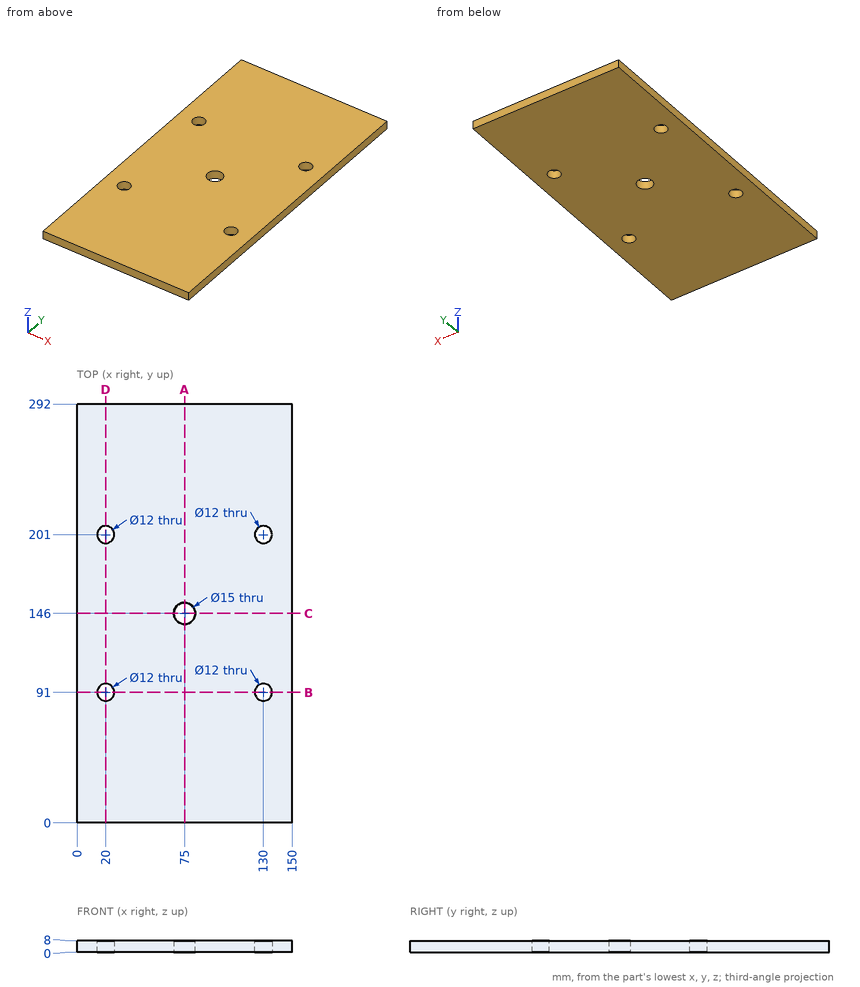
Input: dimensioned drawing with shaded views. Units: mm. Origin: part minimum x, y, z. Coordinates: 2 decimals unless noted, no trailing zeros. Loops run counter-clockwise (first coordinate to the right, second up) from the corner with the lowest first, then second, coordinate; pieces in that order, holes last. Notation, with made-up numbers: (76, -11) -> (106, -11) arc R16 cw to (106, 4) -> close; hole circle Ø10 at (31.25, -12). An arc over 180 degrees is marked (long way). Use a Markdown table: item, result. Add a question column.
(1) Section query B-B, the plane y = 91. Return loops of the section in (x, z), plus the area to 3 significant figures.
(2) Line query: line 1 along Y through (x, z) = (20, 4.5); line 2 along Y through (x, z) = (72, 1). Output: solid intervals per line, ascending.
(3) Section query D-D, the plane x = 20. Return loops of the section in (y, z), plus the area to 3 significant figures.
(4) Section query A-A, the plane x = 75. Return loops of the section in (y, z), plus the area to 3 significant figures.
(5) Section query C-C, the plane y = 146. Return loops of the section in (x, z).
(6) Pin query (flat end, axial travel): pin 1 Ø11 at (x, y) = (130, 91) entering from +Z. Return the tip coordinate at first contact, or that it passes through.
Answer:
| question | item | result |
|---|---|---|
| 1 | outline | (0, 0) -> (14, 0) -> (14, 8) -> (0, 8) -> close; (26, 0) -> (124, 0) -> (124, 8) -> (26, 8) -> close; (136, 0) -> (150, 0) -> (150, 8) -> (136, 8) -> close |
| 1 | area | 1,010 mm^2 |
| 2 | line 1 | y = 0 to 85, 97 to 195, 207 to 292 |
| 2 | line 2 | y = 0 to 139.13, 152.87 to 292 |
| 3 | outline | (0, 0) -> (85, 0) -> (85, 8) -> (0, 8) -> close; (97, 0) -> (195, 0) -> (195, 8) -> (97, 8) -> close; (207, 0) -> (292, 0) -> (292, 8) -> (207, 8) -> close |
| 3 | area | 2,140 mm^2 |
| 4 | outline | (0, 0) -> (138.5, 0) -> (138.5, 8) -> (0, 8) -> close; (153.5, 0) -> (292, 0) -> (292, 8) -> (153.5, 8) -> close |
| 4 | area | 2,220 mm^2 |
| 5 | outline | (0, 0) -> (67.5, 0) -> (67.5, 8) -> (0, 8) -> close; (82.5, 0) -> (150, 0) -> (150, 8) -> (82.5, 8) -> close |
| 6 | pin 1 | passes through |
